```python
from build123d import *

# Parameters (mm, degrees)
SKETCH2_W           = 30
SKETCH2_H           = 17
BOSS_EXTRUDE1_DEPTH = 37
SKETCH3_R           = 6
CUT_EXTRUDE1_DEPTH  = 5.5
CUT_EXTRUDE3_REACH  = 54.479
SKETCH4_R           = 1.5
BOSS_EXTRUDE2_REACH = 52.14
FILLET1_R           = 1


with BuildPart() as part:
    # Sketch2 → Boss-Extrude1 (new body)
    with BuildSketch(Plane(origin=(0, 0, 0), x_dir=(0, 0, -1), z_dir=(1, 0, 0))):
        Polygon((19, -14), (3.999996995, -14), (0, -17.999996995), (-3.999996995, -14), (-19, -14), (-19, 14), (19, 14), align=None)
        Rectangle(SKETCH2_W, SKETCH2_H, mode=Mode.SUBTRACT)
    extrude(amount=BOSS_EXTRUDE1_DEPTH)

    # Sketch3 → Cut-Extrude1 (cut)
    with BuildSketch(Plane(origin=(0, 14, 0), x_dir=(1, 0, 0), z_dir=(0, 1, 0))):
        with Locations(Location((11.5, 0, 0), (0, 0, 270))):
            Circle(SKETCH3_R)
    extrude(amount=-CUT_EXTRUDE1_DEPTH, mode=Mode.SUBTRACT)

    # Sketch4 → Cut-Extrude3 (cut, up to next)
    with BuildSketch(Plane(origin=(0, 14, 0), x_dir=(1, 0, 0), z_dir=(0, 1, 0)), mode=Mode.PRIVATE) as cut_extrude3_sk1:
        with Locations(Location((5.076606241, 7.75, 0), (0, 0, 270))):
            Circle(SKETCH4_R)
    cut_extrude3_tool1 = extrude(cut_extrude3_sk1.sketch, amount=-CUT_EXTRUDE3_REACH, mode=Mode.PRIVATE) & part.part
    # Sketch4 → Cut-Extrude3 (cut, up to next)
    with BuildSketch(Plane(origin=(0, 14, 0), x_dir=(1, 0, 0), z_dir=(0, 1, 0)), mode=Mode.PRIVATE) as cut_extrude3_sk2:
        with Locations(Location((31.923393759, 7.75, 0), (0, 0, 270))):
            Circle(SKETCH4_R)
    cut_extrude3_tool2 = extrude(cut_extrude3_sk2.sketch, amount=-CUT_EXTRUDE3_REACH, mode=Mode.PRIVATE) & part.part
    # Sketch4 → Cut-Extrude3 (cut, up to next)
    with BuildSketch(Plane(origin=(0, 14, 0), x_dir=(1, 0, 0), z_dir=(0, 1, 0)), mode=Mode.PRIVATE) as cut_extrude3_sk3:
        with Locations(Location((31.923393759, -7.75, 0), (0, 0, 270))):
            Circle(SKETCH4_R)
    cut_extrude3_tool3 = extrude(cut_extrude3_sk3.sketch, amount=-CUT_EXTRUDE3_REACH, mode=Mode.PRIVATE) & part.part
    # Sketch4 → Cut-Extrude3 (cut, up to next)
    with BuildSketch(Plane(origin=(0, 14, 0), x_dir=(1, 0, 0), z_dir=(0, 1, 0)), mode=Mode.PRIVATE) as cut_extrude3_sk4:
        with Locations(Location((5.076606241, -7.75, 0), (0, 0, 270))):
            Circle(SKETCH4_R)
    cut_extrude3_tool4 = extrude(cut_extrude3_sk4.sketch, amount=-CUT_EXTRUDE3_REACH, mode=Mode.PRIVATE) & part.part
    add(cut_extrude3_tool1.solids().sort_by_distance((5.076606, 14, -7.75))[0], mode=Mode.SUBTRACT)
    add(cut_extrude3_tool2.solids().sort_by_distance((31.923394, 14, -7.75))[0], mode=Mode.SUBTRACT)
    add(cut_extrude3_tool3.solids().sort_by_distance((31.923394, 14, 7.75))[0], mode=Mode.SUBTRACT)
    add(cut_extrude3_tool4.solids().sort_by_distance((5.076606, 14, 7.75))[0], mode=Mode.SUBTRACT)

    # Boss-Extrude2: up to this face of the body (flat: up to its plane)
    boss_extrude2_end = Plane(part.part.faces().sort_by_distance((19.126018989, 14, 0))[0])
    # Sketch6 → Boss-Extrude2 (add, up to the picked face)
    with BuildSketch(Plane(origin=(0, -14, 0), x_dir=(1, 0, 0), z_dir=(0, 1, 0)), mode=Mode.PRIVATE) as boss_extrude2_sk1:
        with BuildLine():
            Line((47, 3.6), (46.5, 3.6))
            Line((46.5, 3.6), (46.5, 3.1))
            Line((46.5, 3.1), (45.2, 3.1))
            Line((45.2, 3.1), (45.2, 5.5))
            Line((45.2, 5.5), (43.560660172, 5.5))
            Line((43.560660172, 5.5), (41.485786438, 3.425126266))
            ThreePointArc((41.485786438, 3.425126266), (41.052240935, 2.776279568), (40.9, 2.010912703))
            Line((40.9, 2.010912703), (40.9, -2.010912703))
            ThreePointArc((40.9, -2.010912703), (41.052240935, -2.776279568), (41.485786438, -3.425126266))
            Line((41.485786438, -3.425126266), (43.560660172, -5.5))
            Line((43.560660172, -5.5), (45.2, -5.5))
            Line((45.2, -5.5), (45.2, -3.1))
            Line((45.2, -3.1), (46.5, -3.1))
            Line((46.5, -3.1), (46.5, -3.6))
            Line((46.5, -3.6), (47, -3.6))
            Line((47, -3.6), (47, -10))
            Line((47, -10), (37, -10))
            Line((37, -10), (37, 10))
            Line((37, 10), (47, 10))
            Line((47, 10), (47, 3.6))
        make_face()
    boss_extrude2_tool1 = split(extrude(boss_extrude2_sk1.sketch, amount=BOSS_EXTRUDE2_REACH, mode=Mode.PRIVATE), bisect_by=boss_extrude2_end, keep=Keep.BOTH, mode=Mode.PRIVATE)
    add(boss_extrude2_tool1.solids().sort_by(Axis((46.75, -14, -3.823607), (0, 1, 0)))[0])

    # Fillet1
    fillet1_edges = [part.edges().sort_by_distance(p)[0] for p in [
        (42, 14, -10),
        (0, -8.5, 0),
        (0, 0, 15),
        (0, 8.5, 0),
        (0, 0, -15),
        (0, -14, 11.499998498),
        (0, -15.999998498, 1.999998498),
        (0, -15.999998498, -1.999998498),
        (0, -14, -11.499998498),
        (0, 14, 0),
        (18.5, -14, -19),
        (37, 0, -19),
        (18.5, 14, -19),
        (0, 0, -19),
        (18.5, 14, 19),
        (37, 0, 19),
        (18.5, -14, 19),
        (0, 0, 19),
        (37, 14, -14.5),
        (37, 11.25, -10),
        (42, 14, 10),
        (37, 14, 14.5),
        (47, 0, -10),
        (47, 0, 10),
        (47, 14, 6.8),
        (47, -14, 6.8),
        (47, 14, -6.8),
        (47, -14, -6.8),
    ]]
    fillet(fillet1_edges, radius=FILLET1_R)


solid = part.part
```
Can you work these out from the model? Positions are in its coordinate system, mm. A direction names the side the tool comes from. Round coordinates to 2 decimals unless told otherwise and drop trailing zeros. Order: outer loops, then holes, each group sorted by start corner. A loop starts at its lowest first (then second) coordinate and runs counter-clockwise, first axis right, second up. Notation, with made-up numbers: (-12.5, 73) -> (44.5, 73) arc R21 ccw to (44.5, 87) -> close; hole circle Ø9 at (70, 76). An arc over 180 degrees is marked (long way). Return JSON: item names as keys, results as strings. Group by question number.
1. We'd pull the mould along X, two halves only. Please class faces 5 (the face through (46, 0, 3.1)), 6 (the face through (42.54, -0.2, -4.48)), 7 (the face through (37, 0, -16)): released by +X, released by -X, zero draft, split by the parting line, or undercut.
2. If we section it at D-D, the plane x = 11.5: Write out the boundary of the cut face in (y, z), then the cut area to 3 significant figures.
3. Which directions (+Z, -Z, +X, -X, +Y, -Y) give clear straight access to the entire face, cutting with the end or side of a thin tool? Please do faces 1 (the face through (45.2, 0, 4)), 2 (the face through (19, 0, 15)), 3 (the face through (33.41, 11.29, 7.55)), 4 (the face through (37, 0, 16)).
4. If we section it at C-C, the plane z = 17: Write out the boundary of the cut face in (x, y).
5. If we section it at A-A, the plane x = 35: Write out the boundary of the cut face in (y, z).
6. Will these pins go through, and if not, where does the flat tip stop? pin 1 (3 mm diameter, centred on y = 10.5, z = 0.5, fed in from +X); pin 2 (0.5 mm diameter, centred on x = 45, y = -4, fed in from +Z); pin 3 (1.8 mm diameter, centred on x = 31.92, z = -7.75, fed in from +Y).
7. If we section it at B-B, the plane z = -8: Write out the boundary of the cut face in (x, y).
8. I need wall thicknesses on line 1 (X direction, y = 10.15, z = -7.75); line 2 (Z direction, x = 45, y = -10); line 3 (Y direction, x = 11, z = -12.5). Which ranges of each line are inside material? Lowest first, please. Write a range as [from, to].
Output values:
{
 "1": {"face 5": "zero draft", "face 6": "undercut", "face 7": "released by +X"},
 "2": {"outline": "(-18, 0) -> (-14, -4) -> (-14, -18) arc R1 ccw to (-13, -19) -> (13, -19) arc R1 ccw to (14, -18) -> (14, -6) -> (8.5, -6) -> (8.5, -15) -> (-8.5, -15) -> (-8.5, 15) -> (8.5, 15) -> (8.5, 6) -> (14, 6) -> (14, 18) arc R1 ccw to (13, 19) -> (-13, 19) arc R1 ccw to (-14, 18) -> (-14, 4) -> close", "area": "503 mm²"},
 "3": {"face 1": "+Y, -Y", "face 2": "+X, -X", "face 3": "+Y", "face 4": "+Z, +X, +Y, -Y"},
 "4": {"outline": "(0, -13) arc R1 ccw to (1, -14) -> (37, -14) -> (37, 13) arc R1 ccw to (36, 14) -> (1, 14) arc R1 ccw to (0, 13) -> close"},
 "5": {"outline": "(-18, 0) -> (-14, -4) -> (-14, -18) arc R1 ccw to (-13, -19) -> (13, -19) arc R1 ccw to (14, -18) -> (14, 18) arc R1 ccw to (13, 19) -> (-13, 19) arc R1 ccw to (-14, 18) -> (-14, 4) -> close; hole (-8.5, -15) -> (8.5, -15) -> (8.5, 15) -> (-8.5, 15) -> close"},
 "6": {"pin 1": "x = 40.9", "pin 2": "z = 10", "pin 3": "y = -8.5"},
 "7": {"outline": "(0, -13) arc R1 ccw to (1, -14) -> (46, -14) arc R1 ccw to (47, -13) -> (47, 13) arc R1 ccw to (46, 14) -> (33.4, 14) -> (33.4, 8.5) -> (37, 8.5) -> (37, -8.5) -> (1, -8.5) arc R1 ccw to (0, -9.5) -> close; (0, 9.5) arc R1 ccw to (1, 8.5) -> (3.6, 8.5) -> (3.6, 14) -> (1, 14) arc R1 ccw to (0, 13) -> close; (6.56, 8.5) -> (30.44, 8.5) -> (30.44, 14) -> (6.56, 14) -> close"},
 "8": {"line 1": "[0, 3.58], [6.58, 30.42], [33.42, 47]", "line 2": "[-10, -5.5], [5.5, 10]", "line 3": "[-14, -8.5], [8.5, 14]"}
}
